```python
from build123d import *

# Parameters (mm, degrees)
SKETCH_R     = 1.725
PAD_DEPTH    = 2.5
SKETCH002_W  = 3
SKETCH002_H  = 7
PAD001_DEPTH = 8
SKETCH003_W  = 14
SKETCH003_H  = 7
SKETCH003_R  = 2.1
PAD002_DEPTH = 2


with BuildPart() as part:
    # Sketch → Pad (new body)
    with BuildSketch(Plane.XY):
        with BuildLine():
            Line((-19.96, -19), (-11.96, -19))
            Line((-11.96, -19), (-11.96, -15))
            Line((-11.96, -15), (-11.646424, -13.789971))
            ThreePointArc((-5.5, 17.19164), (-17.704944, 3.512474), (-11.646424, -13.789971))
            Line((-5.5, 21.5), (-5.5, 17.19164))
            Line((-5.5, 21.5), (5.5, 21.5))
            Line((5.5, 21.5), (5.5, 17.19164))
            ThreePointArc((11.646424, -13.789971), (17.704944, 3.512474), (5.5, 17.19164))
            Line((11.96, -15), (11.646424, -13.789971))
            Line((11.96, -19), (11.96, -15))
            Line((11.96, -19), (20.04, -19))
            Line((20.04, -19), (25.96, -19))
            Line((25.96, -19), (25.96, 26))
            Line((25.96, 26), (20, 26))
            Line((-20, 26), (20, 26))
            Line((-20, 26), (-25.96, 26))
            Line((-25.96, 26), (-25.96, -19))
            Line((-19.96, -19), (-25.96, -19))
        make_face()
        with Locations((-14.96, 15)):
            Circle(SKETCH_R, mode=Mode.SUBTRACT)
        with Locations((15, 15)):
            Circle(SKETCH_R, mode=Mode.SUBTRACT)
        with Locations((-14.96, -15)):
            Circle(SKETCH_R, mode=Mode.SUBTRACT)
        with Locations((15, -15)):
            Circle(SKETCH_R, mode=Mode.SUBTRACT)
    extrude(amount=PAD_DEPTH)

    # Sketch002 (on Face24 of Pad) → Pad001 (join)
    with BuildSketch(Plane.XY.offset(2.5)):
        with Locations((-24.46, 22.5)):
            Rectangle(SKETCH002_W, SKETCH002_H)
        with Locations((-24.46, -15.5)):
            Rectangle(SKETCH002_W, SKETCH002_H)
        with Locations((24.46, -15.5)):
            Rectangle(SKETCH002_W, SKETCH002_H)
        with Locations((24.46, 22.5)):
            Rectangle(SKETCH002_W, SKETCH002_H)
    extrude(amount=PAD001_DEPTH)

    # Sketch003 (on Face25 of Pad001) → Pad002 (join)
    with BuildSketch(Plane.XY.offset(10.5)):
        with Locations((-29.96, 22.5)):
            Rectangle(SKETCH003_W, SKETCH003_H)
        with Locations((-32.96, 22.5)):
            Circle(SKETCH003_R, mode=Mode.SUBTRACT)
        with Locations((-29.96, -15.5)):
            Rectangle(SKETCH003_W, SKETCH003_H)
        with Locations((-32.96, -15.5)):
            Circle(SKETCH003_R, mode=Mode.SUBTRACT)
        with Locations((29.96, -15.5)):
            Rectangle(SKETCH003_W, SKETCH003_H)
        with Locations((32.96, -15.5)):
            Circle(SKETCH003_R, mode=Mode.SUBTRACT)
        with Locations((29.96, 22.5)):
            Rectangle(SKETCH003_W, SKETCH003_H)
        with Locations((32.96, 22.5)):
            Circle(SKETCH003_R, mode=Mode.SUBTRACT)
    extrude(amount=PAD002_DEPTH)


solid = part.part
```
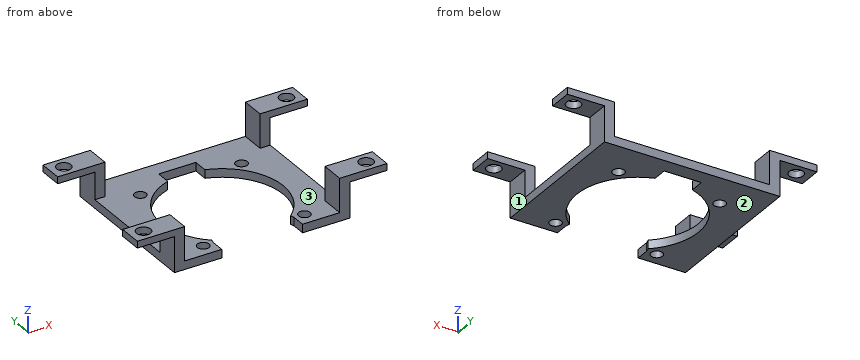
For this review, take the finished solid that the model builds, in its own axes (mm). Face numbers are marked on the shaded views. Give positions to 0.01 mm unless a question says otherwise; leave off trailing zeros. Write each loop counter-clockwise with the first axis right and the second up, starting at its lowest first coordinate (ties: lowest second). Pieces come first, ordered by that corner, then holes. Notation, with made-up numbers: M 52,-16.75 L 69,-16.75 A6 cw 69,-7.75 Z; hole C 20,60.5 d6. An arc over 180 degrees is marked long. Answer as a JSON object with one key per item and string values. Group by question number.
Item 1: Consider section C-C on z = 5. Write out the cut boundary in (x, y), plus the area to 3 significant figures.
Item 2: Draft analysis for pull direction X (two halves, no side actions). For the marked faces 1, 2 and 3, state which applies: +X half, -X half, draft (parallel to the pull), parting line (faces both ways), or undercut.
Item 3: Consider section B-B on x = -32.96. Write out the cut boundary in (y, z).
Item 4: For probe 1 along X at (y, z) = (16.5, 1.25); probe 2 along Y at (x, z) = (15, 1.1) (3 decimals); probe 3 along X at (y, z) = (22.5, 8), list the stretches that pass through material, from the lowest coordinate up. Write a range as [from, to].
Item 5: For pin 1 Ø2 at (y, z) = (19.5, 1.5) entering from -X; pin 2 Ø4 at (x, y) = (-14.96, -15) entering from +Z; pin 3 Ø5 at (x, y) = (-32.96, 22.5) entering from -Z, all flat-tipped, find the tip position at first contact; note any pin that passes through.
Item 6: Consider section D-D on y = 22.5. Write out the cut boundary in (x, z), plus the area to 3 significant figures.
Item 7: Consider section A-A on z = 11.5. Write out the cut boundary in (x, y).
Check result:
{
 "1": {"outline": "M -25.96,-19 L -22.96,-19 L -22.96,-12 L -25.96,-12 Z; M -25.96,19 L -22.96,19 L -22.96,26 L -25.96,26 Z; M 22.96,-19 L 25.96,-19 L 25.96,-12 L 22.96,-12 Z; M 22.96,19 L 25.96,19 L 25.96,26 L 22.96,26 Z", "area": "84.0 mm^2"},
 "2": {"face 1": "+X half", "face 2": "draft", "face 3": "undercut"},
 "3": {"outline": "M -19,10.5 L -17.6,10.5 L -17.6,12.5 L -19,12.5 Z; M -13.4,10.5 L -12,10.5 L -12,12.5 L -13.4,12.5 Z; M 19,10.5 L 20.4,10.5 L 20.4,12.5 L 19,12.5 Z; M 24.6,10.5 L 26,10.5 L 26,12.5 L 24.6,12.5 Z"},
 "4": {"probe 1": "x = [-25.96, -15.81], [-14.11, -7.32], [7.32, 14.15], [15.85, 25.96]", "probe 2": "y = [-19, -16.725], [-13.275, -10.04], [10.04, 13.275], [16.725, 26]", "probe 3": "x = [-25.96, -22.96], [22.96, 25.96]"},
 "5": {"pin 1": "stops at x = -25.96", "pin 2": "stops at z = 2.5", "pin 3": "stops at z = 10.5"},
 "6": {"outline": "M -36.96,10.5 L -35.06,10.5 L -35.06,12.5 L -36.96,12.5 Z; M -30.86,10.5 L -25.96,10.5 L -25.96,0 L 25.96,0 L 25.96,10.5 L 30.86,10.5 L 30.86,12.5 L 22.96,12.5 L 22.96,2.5 L -22.96,2.5 L -22.96,12.5 L -30.86,12.5 Z; M 35.06,10.5 L 36.96,10.5 L 36.96,12.5 L 35.06,12.5 Z", "area": "217 mm^2"},
 "7": {"outline": "M -36.96,-19 L -22.96,-19 L -22.96,-12 L -36.96,-12 Z; M -36.96,19 L -22.96,19 L -22.96,26 L -36.96,26 Z; M 22.96,-19 L 36.96,-19 L 36.96,-12 L 22.96,-12 Z; M 22.96,19 L 36.96,19 L 36.96,26 L 22.96,26 Z; hole C -32.96,-15.5 d4.2; hole C -32.96,22.5 d4.2; hole C 32.96,-15.5 d4.2; hole C 32.96,22.5 d4.2"}
}
